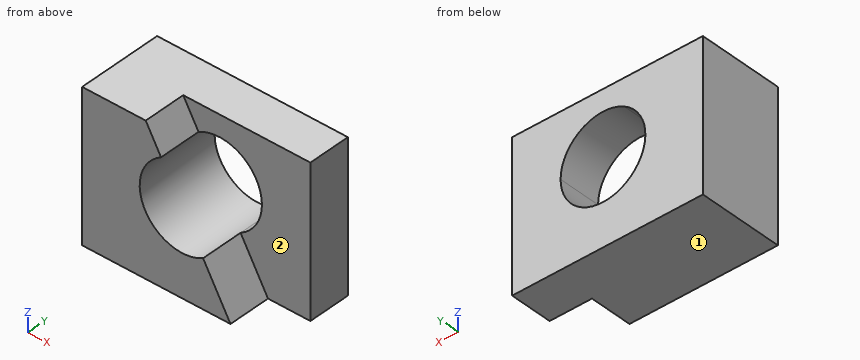
```python
from build123d import *

# Parameters (mm, degrees)
F0_W     = 114.3
F0_H     = 88.9
F1_DEPTH = 25.4
F3_DEPTH = 25.4
F5_DEPTH = 50.8


with BuildPart() as f1:
    # F0 (on Front) → F1 (new body)
    with BuildSketch(Plane.XZ):
        with Locations((11.960601, 7.462785)):
            Rectangle(F0_W, F0_H)
    extrude(amount=F1_DEPTH)

    # F2 (on face) → F3 (join)
    with BuildSketch(Plane.XZ.offset(25.4)):
        Polygon((-45.189399, 51.912785), (-45.189399, -36.987215), (43.710601, -36.987215), (-7.089399, 51.912785), align=None)
    extrude(amount=F3_DEPTH)

    # F4 (on face) → F5 (cut)
    with BuildSketch(Plane.XZ.offset(50.8)):
        with BuildLine():
            ThreePointArc((27.283958, -8.240591), (36.650746, 1.063844), (40.082029, 13.812785))
            ThreePointArc((40.082029, 13.812785), (27.43097, 35.781501), (2.0801, 35.866161))
            Line((2.0801, 35.866161), (27.283958, -8.240591))
        make_face()
        with BuildLine():
            Line((27.283958, -8.240591), (2.0801, 35.866161))
            ThreePointArc((2.0801, 35.866161), (-7.371347, 1.210856), (27.283958, -8.240591))
        make_face()
    extrude(amount=-F5_DEPTH, mode=Mode.SUBTRACT)


solid = f1.part
```
CAD build for the part. Positions are in the model's coordinates, mm. Face numbers are marked on the shaded views. A direction names the side the tool comes from. Round coordinates to 2 decimals unless told otherwise and drop trailing zeros. Order: outer loops, then holes, each group sorted by start corner. A loop starts at its lowest first (then second) coordinate and runs counter-clockwise, first axis right, second up.
Q1. Slice it at A-A (y = -11). Write the cut outline in (x, z).
Q2. Slice it at B-B (x = 35). Write the cut outline in (y, z), and give its area (3 significant figures).
Q3. Wall check: L1, parallel to X at y = -11, z = 13.5; L2, parallel to Y at x = 40, z = -26.5; L3, parallel to X at y = -29, z = 14. Give the ranges that are in metal, low to high.
Q4. Slice it at C-C (z = 34.5). Write the cut outline in (x, y).
Q5. Drop flat-ended pins along their axis: pin 1 (2 mm diameter, centred on y = -33.5, z = 5.5, fed in from +X); pin 2 (10 mm diameter, centred on x = 40.5, y = -33.5, fed in from +Z); pin 3 (1 mm diameter, centred on y = -42, z = 4.5, fed in from +X). Give the stop position or say it passes through.
Q6. Which spindle directions (+Z, -Z, +X, -X, +Y, -Y) get a long thin tool onto all of the face, cutting with end or side? Do the marked faces 1 and 2. Say none if no direction does.
Q7. Slice it at D-D (y = -27). Write the cut outline in (x, z), and give its area (3 significant figures).
Results below:
1. outline: (-45.19, -36.99) - (69.11, -36.99) - (69.11, 51.91) - (-45.19, 51.91) - close; hole (27.28, -8.24) arc R25.4 ccw to (40.08, 13.81) arc R25.4 ccw (long way) to start
2. outline: (-50.8, -36.99) - (0, -36.99) - (0, -1.43) - (-25.4, -1.43) - (-25.4, -21.74) - (-50.8, -21.74) - close; (-25.4, 29.06) - (0, 29.06) - (0, 51.91) - (-25.4, 51.91) - close
2. area: 1,870 mm2
3. L1: x = -45.19 to -10.72, 40.08 to 69.11
3. L2: y = -25.4 to 0
3. L3: x = -45.19 to -10.72
4. outline: (-45.19, -50.8) - (-0.06, -50.8) - (-0.06, 0) - (-45.19, 0) - close; (29.42, -25.4) - (69.11, -25.4) - (69.11, 0) - (29.42, 0) - close
5. pin 1: stops at x = -8.95
5. pin 2: stops at z = -22.62
5. pin 3: stops at x = -8.75
6. face 1: -Z, +X, -X, +Y, -Y
6. face 2: +Z, +X, -Y
7. outline: (-45.19, -36.99) - (43.71, -36.99) - (27.28, -8.24) arc R25.4 cw to (2.08, 35.87) - (-7.09, 51.91) - (-45.19, 51.91) - close
7. area: 4,630 mm2
